The figure shows three views and two pictorial views of one solid part (mm, origin at its lowest corner). Answer the questions. Coordinates: 2 decimals unless noted, no trailing zeros. Write each loop counter-clockwise with the first axis right and the second up, starting at its lowest first coordinate (ties: lowest second). Pieces come first, ordered by that corner, then holes. Notation, with made-up numbers: M 65,53.25 L 103,53.25 A32 cw 103,81.25 Z; hole C 72.5,48.25 d2. An arc over 180 degrees is marked long. Answer as CSV lines item,"result".
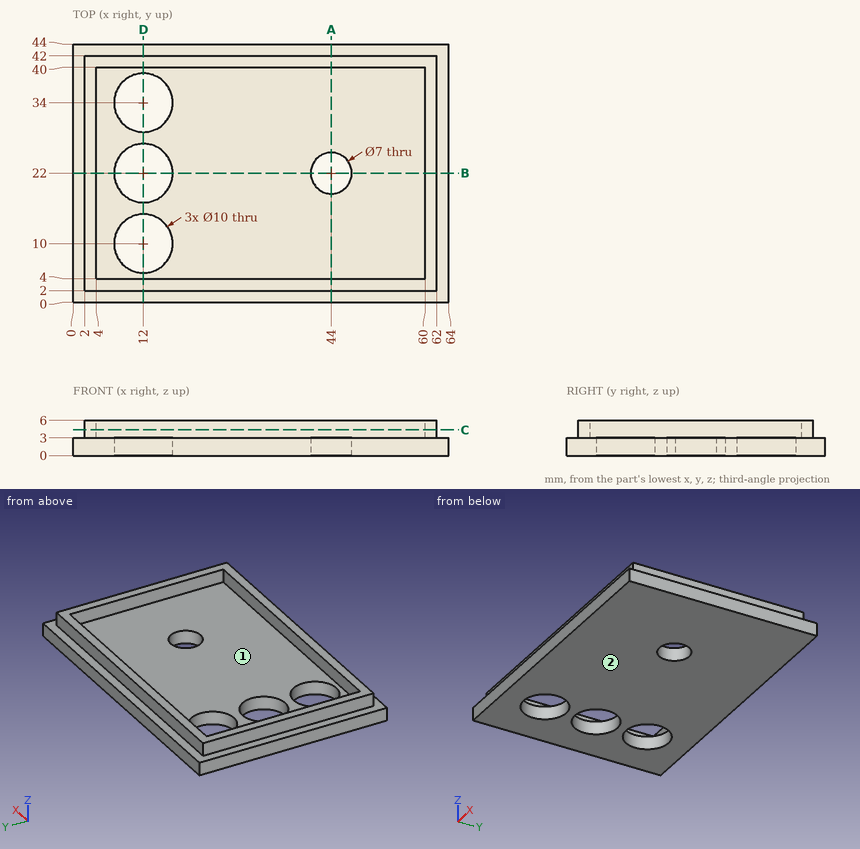
Q1. Straight lines are drawn through the part: line 1 (Y direction, x = 12, z = 1.05); line 2 (Y direction, x = 44, z = 0.9); line 3 (Y direction, x = 17, z = 5.4). For each, find the intervals that lie inside material, in ascending order.
Output:
line 1,"0 to 5, 15 to 17, 27 to 29, 39 to 44"
line 2,"0 to 18.5, 25.5 to 44"
line 3,"2 to 4, 40 to 42"
Q2. Find section A-A (x = 44). Give the vertices of the cut face in (y, z).
Output:
outline,"M 0,0 L 18.5,0 L 18.5,3 L 4,3 L 4,6 L 2,6 L 2,3 L 0,3 Z; M 25.5,0 L 44,0 L 44,3 L 42,3 L 42,6 L 40,6 L 40,3 L 25.5,3 Z"
Q3. The mould has two halves that part along X. Classify the marked faces 1 and 2: pulls with the +X half, pulls with the -X half, needs draft (parallel to the pull), parting line crosses it, or undercut.
Output:
face 1,"undercut"
face 2,"needs draft"
Q4. Find section C-C (z = 4.35). Give the vertices of the cut face in (x, y).
Output:
outline,"M 2,2 L 62,2 L 62,42 L 2,42 Z; hole M 4,4 L 60,4 L 60,40 L 4,40 Z"
Q5. Find section D-D (x = 12). Give the vertices of the cut face in (y, z).
Output:
outline,"M 0,0 L 5,0 L 5,3 L 4,3 L 4,6 L 2,6 L 2,3 L 0,3 Z; M 15,0 L 17,0 L 17,3 L 15,3 Z; M 27,0 L 29,0 L 29,3 L 27,3 Z; M 39,0 L 44,0 L 44,3 L 42,3 L 42,6 L 40,6 L 40,3 L 39,3 Z"
Q6. Find section B-B (y = 22). Give the vertices of the cut face in (x, z).
Output:
outline,"M 0,0 L 7,0 L 7,3 L 4,3 L 4,6 L 2,6 L 2,3 L 0,3 Z; M 17,0 L 40.5,0 L 40.5,3 L 17,3 Z; M 47.5,0 L 64,0 L 64,3 L 62,3 L 62,6 L 60,6 L 60,3 L 47.5,3 Z"
Q7. Flat-ended cylindrical pins translate along their axes: pin 1 Ø0.9 at (y, z) = (13.5, 4.5) entering from -X; pin 2 Ø1.5 at (x, z) = (43, 5) entering from -Y; pin 3 Ø11 at (x, y) = (31, 20.5) entering from +Z. Find the tip coordinate at first contact, or state that the pin passes through.
Output:
pin 1,"x = 2"
pin 2,"y = 2"
pin 3,"z = 3"
